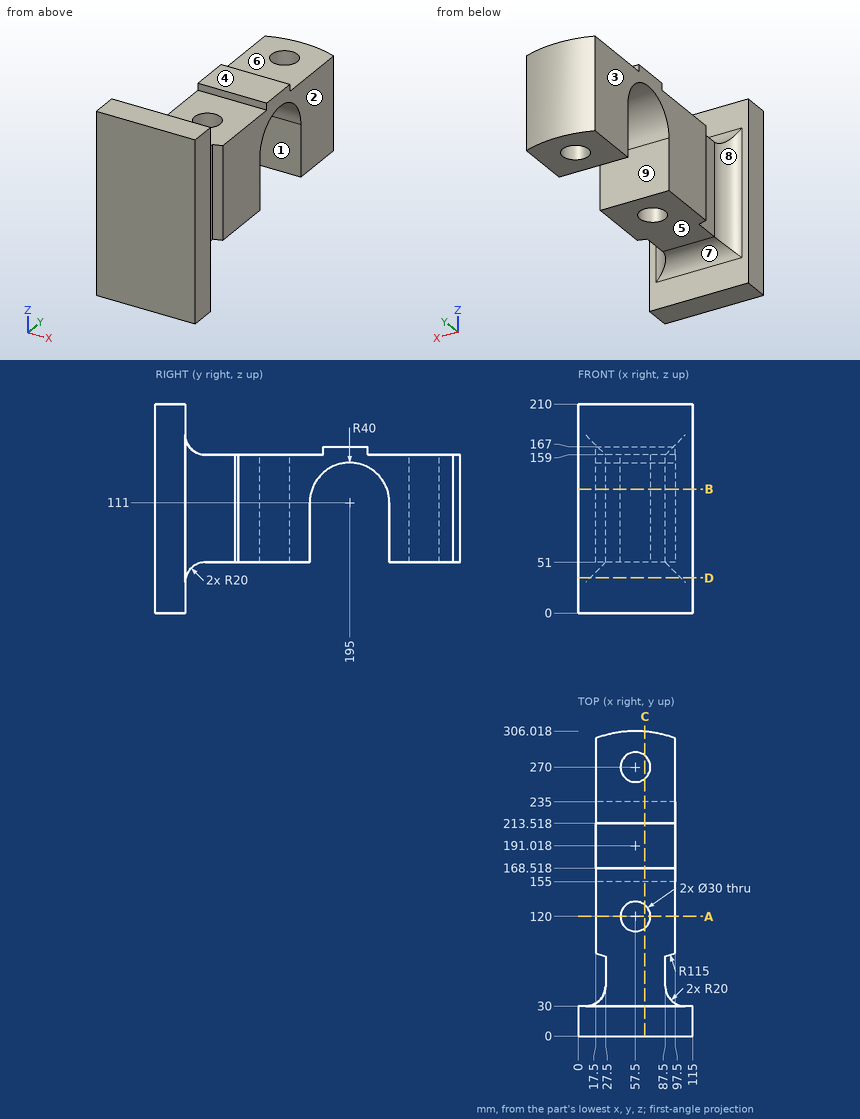
Study the drawing (mm; zero at the part's minimum x, y, z) and answer. A direction names the side the tool comes from. Coordinates: 2 decimals unless noted, no trailing zeros. Write each loop counter-clockwise with the first axis right and the second up, starting at its lowest first coordinate (ties: lowest second). Pieces come first, ordered by that corner, then holes. Notation, with made-up numbers: (-9.75, 71.25) - (11.25, 71.25) arc R13 cw to (11.25, 76.25) - close; hole circle Ø5 at (29.25, 17). An arc over 180 degrees is marked (long way). One line per item, written item: value.
1) Find section C-C (x = 67). Give the vertices of the cut face in (y, z), and give its area (3 significant figures).
Geometry check:
outline: (0, 0) - (30, 0) - (30, 31) arc R20 cw to (50, 51) - (108.39, 51) - (108.39, 159) - (50, 159) arc R20 cw to (30, 179) - (30, 210) - (0, 210) - close; (131.61, 51) - (155, 51) - (155, 111) arc R40 cw to (235, 111) - (235, 51) - (258.39, 51) - (258.39, 159) - (213.52, 159) - (213.52, 167) - (168.52, 167) - (168.52, 159) - (131.61, 159) - close; (281.61, 51) - (305.62, 51) - (305.62, 159) - (281.61, 159) - close
area: 24,300 mm2
2) Find section B-B (z = 124.5). Give the vertices of the cut face in (x, y).
Geometry check:
outline: (0, 0) - (115, 0) - (115, 30) - (107.5, 30) arc R20 cw to (87.5, 50) - (87.5, 80) arc R115 ccw to (97.5, 83.2) - (97.5, 157.35) - (17.5, 157.35) - (17.5, 83.2) arc R115 ccw to (27.5, 80) - (27.5, 50) arc R20 cw to (7.5, 30) - (0, 30) - close; (17.5, 232.65) - (97.5, 232.65) - (97.5, 298.84) arc R115 ccw to (17.5, 298.84) - close; hole circle Ø30 at (57.5, 120); hole circle Ø30 at (57.5, 270)
3) A tool of negligible diameter and unlimited length cuts with its end or side. For the marked faces 1, 2, 3, 4 and 5, from which of +Z, -Z, +X, -X, +Y, -Y can it reach the whole face along a straight path? Write none if from no direction.
Geometry check:
face 1: -Z, +X, -X
face 2: +Z, -Z, +X, +Y
face 3: +Z, -Z, -X, +Y
face 4: +Z, +X, -X, +Y
face 5: -Z, +X, -X, +Y
4) Find section D-D (z = 35.5). Give the vertices of the cut face in (x, y), and give its area (3 significant figures).
Geometry check:
outline: (0, 0) - (115, 0) - (115, 30) - (107.5, 30) arc R20 cw to (103, 30.51) - (12, 30.51) arc R20 cw to (7.5, 30) - (0, 30) - close
area: 3,500 mm2
5) Consider line 1 along Y through (x, z) = (57.5, 113); line 2 along Y through (x, z) = (57.5, 73); line 3 along Y through (x, z) = (89.5, 93.5). Determine where each line is inside the solid, lowest interval first. Write a range as from..to.
Geometry check:
line 1: y = 0..105, 135..155.05, 234.95..255, 285..306.02
line 2: y = 0..105, 135..155, 235..255, 285..306.02
line 3: y = 0..41.28, 80.56..155, 235..301.48
6) Find section A-A (y = 120). Give the vertices of the cut face in (x, z), and give its area (3 significant figures).
Geometry check:
outline: (17.5, 51) - (42.5, 51) - (42.5, 159) - (17.5, 159) - close; (72.5, 51) - (97.5, 51) - (97.5, 159) - (72.5, 159) - close
area: 5,400 mm2
7) For a pull along Y with two mould halves and no side action, classify the marked faces 6, 7, 8 and 9 as pulls with the +Y half, pulls with the -Y half, needs draft (parallel to the pull), parting line crosses it, or undercut.
Geometry check:
face 6: needs draft
face 7: pulls with the +Y half
face 8: undercut
face 9: undercut
8) Each of these flat-tipped pins is pushed along its axis until it touches: pin 1 Ø5 at (x, y) = (97, 244) entering from +Z; pin 2 Ø12 at (x, z) = (90, 82) entering from +Y; pin 3 Ø1 at (x, z) = (64.5, 184.5) entering from +Y. Where does it stop, or does it pass through?
Geometry check:
pin 1: stops at z = 159
pin 2: stops at y = 302.92
pin 3: stops at y = 30
